Source: CAD feature listing. Evaluate the final solid. Frame: model axes, mm. A direction names the side the tool comes from. Coordinates: 2 decimals unless noted, no trailing zeros. Write each loop counter-clockwise with the first axis right and the second up, starting at its lowest first coordinate (ties: lowest second). Pieces come first, ordered by that corner, then holes. Notation, with made-up numbers: (3.5, 64.5) - (7.5, 64.5) arc R15 cw to (7.5, 78.5) - close; hole circle Ø5 at (-6.75, -15.75). An arc over 180 degrees is marked (long way). One line per question, with ' | ' between items. Start each with the question number.
Q1. Contact query for flat-ended pins moving along their axis: P1, Ø2, axis at x = -22.5, z = 9.5, coming from the -Y side; P2, Ø0.9, axis at x = -8.5, z = -1.5, coming from the +Y side; P3, Ø1.5, axis at x = 22.5, z = -1.5, coming from the -Y side; P4, Ø3.5, axis at x = 4, y = 24, coming from the +Z side. Output: stop coordinate, or through.
Q2. Draft query along X for faces 1 (the face through (-65, 1, -3)), 2 (the face through (-57.09, 12.25, -0.77)). Return one class per face: +X half, -X half, draft (parallel to the pull), parting line (faces both ways), or undercut.
Q3. Cut plane A-A, the plane z = 9. Return loops of the section in (x, y), plus the area to 3 significant figures.
Q4. Cut plane D-D, the plane y = 29. Return loops of the section in (x, z).
Q5. Cut plane B-B, the plane x = 4. Return loops of the section in (y, z).
Q6. Access query for faces 3 (the face through (-5.04, -16.49, -0.77)), 4 (the face through (-168, 0, 2.9)), 5 (the face through (-76.034, 33.187, 16.306)). Directions: +Z, -Z, +X, -X, +Y, -Y. A direction counts if a zero-diameter tool reaches every point of the face in a straight line with its end or side. Return the directions, or none.
Q7. Line query: line 1 (Y direction, x = 4, z = -1.4); line 2 (Y direction, x = 0, z = 24); line 3 (Z direction, x = -48.5, y = -21.5). Output: solid intervals per line, ascending.
Q8. Cut plane C-C, the plane z = 28. Return loops of the section in (x, y), plus the area to 3 significant figures.
```python
from build123d import *

# Parameters (mm, degrees)
ESBO_O1_R                  = 9.95
ESBO_O1_R_2                = 1.9
ESBO_O1_R_3                = 10
ESBO_O1_R_4                = 2.9
RESSALTO_EXTRUS_O1_DEPTH   = 30.8
ESBO_O1_3_R                = 9.95
ESBO_O1_3_R_2              = 1.9
ESBO_O1_3_R_3              = 10
ESBO_O1_3_R_4              = 2.9
RESSALTO_EXTRUS_O2_DEPTH   = 3
RESSALTO_EXTRUS_O4_DEPTH   = 33.8
CORTE_EXTRUS_O1_DEPTH      = 29.4
ESBO_O1_4_R                = 9.95
ESBO_O1_4_R_2              = 1.9
ESBO_O1_4_R_3              = 10
ESBO_O1_4_R_4              = 2.9
CORTE_EXTRUS_O2_DEPTH      = 31.8
CORTE_EXTRUS_O2_DEPTH_BACK = 4
RESSALTO_EXTRUS_O5_DEPTH   = 30.8
FILETE1_R                  = 10
CORTE_EXTRUS_O3_REACH      = 226.029
ESBO_O5_W                  = 22
ESBO_O5_H                  = 6


with BuildPart() as part:
    # Esboço1 → Ressalto-extrusão1 (new body)
    with BuildSketch(Plane.XY):
        with BuildLine():
            Line((-176.929134073, 19.50886441), (-176.929134073, -21.49113559))
            Line((-176.929134073, -21.49113559), (-5.303716409, -42.772427944))
            ThreePointArc((-5.303716409, -42.772427944), (43.09930295, 0.245122927), (-5.789885285, 42.709334207))
            Line((-5.789885285, 42.709334207), (-176.929134073, 19.50886441))
        make_face()
        with Locations((-44.879134073, -0.99113559)):
            Circle(ESBO_O1_R, mode=Mode.SUBTRACT)
        with Locations((-58.844493002, 12.974223338)):
            Circle(ESBO_O1_R_2, mode=Mode.SUBTRACT)
        with Locations((-97.729134073, -0.99113559)):
            Circle(ESBO_O1_R_3, mode=Mode.SUBTRACT)
        with Locations((-58.844493002, -14.956494518)):
            Circle(ESBO_O1_R_2, mode=Mode.SUBTRACT)
        with Locations((4, 24)):
            Circle(ESBO_O1_R_4, mode=Mode.SUBTRACT)
        with BuildLine():
            Line((22.160394843, 16.45886441), (24.010394843, 16.45886441))
            ThreePointArc((24.010394843, 16.45886441), (26.010394843, 14.45886441), (24.010394843, 12.45886441))
            Line((24.010394843, 12.45886441), (22.160394843, 12.45886441))
            ThreePointArc((22.160394843, 12.45886441), (20.160394843, 14.45886441), (22.160394843, 16.45886441))
        make_face(mode=Mode.SUBTRACT)
        with Locations((-30.913775145, -14.956494518)):
            Circle(ESBO_O1_R_2, mode=Mode.SUBTRACT)
        with BuildLine():
            Line((-7.039605157, -18.44113559), (-8.889605157, -18.44113559))
            ThreePointArc((-8.889605157, -18.44113559), (-10.889605157, -16.44113559), (-8.889605157, -14.44113559))
            Line((-8.889605157, -14.44113559), (-7.039605157, -14.44113559))
            ThreePointArc((-7.039605157, -14.44113559), (-5.039605157, -16.44113559), (-7.039605157, -18.44113559))
        make_face(mode=Mode.SUBTRACT)
        with BuildLine():
            Line((24.010394843, -18.44113559), (22.160394843, -18.44113559))
            ThreePointArc((22.160394843, -18.44113559), (20.160394843, -16.44113559), (22.160394843, -14.44113559))
            Line((22.160394843, -14.44113559), (24.010394843, -14.44113559))
            ThreePointArc((24.010394843, -14.44113559), (26.010394843, -16.44113559), (24.010394843, -18.44113559))
        make_face(mode=Mode.SUBTRACT)
        with Locations((-30.913775145, 12.974223338)):
            Circle(ESBO_O1_R_2, mode=Mode.SUBTRACT)
        with BuildLine():
            ThreePointArc((-0.025, -11.375), (-11.4, 0), (-0.025, 11.375))
            Line((-0.025, 11.375), (0.025, 11.375))
            ThreePointArc((0.025, 11.375), (11.4, 0), (0.025, -11.375))
            Line((0.025, -11.375), (-0.025, -11.375))
        make_face(mode=Mode.SUBTRACT)
        with BuildLine():
            ThreePointArc((-8.889605157, 12.45886441), (-10.889605157, 14.45886441), (-8.889605157, 16.45886441))
            Line((-8.889605157, 16.45886441), (-7.039605157, 16.45886441))
            ThreePointArc((-7.039605157, 16.45886441), (-5.039605157, 14.45886441), (-7.039605157, 12.45886441))
            Line((-7.039605157, 12.45886441), (-8.889605157, 12.45886441))
        make_face(mode=Mode.SUBTRACT)
    extrude(amount=RESSALTO_EXTRUS_O1_DEPTH)

    # Esboço1<3> → Ressalto-extrusão2 (add)
    with BuildSketch(Plane.XY):
        with BuildLine():
            Line((-176.929134073, 19.50886441), (-176.929134073, -21.49113559))
            Line((-176.929134073, -21.49113559), (-5.303716409, -42.772427944))
            ThreePointArc((-5.303716409, -42.772427944), (43.09930295, 0.245122927), (-5.789885285, 42.709334207))
            Line((-5.789885285, 42.709334207), (-176.929134073, 19.50886441))
        make_face()
        with Locations((-44.879134073, -0.99113559)):
            Circle(ESBO_O1_3_R, mode=Mode.SUBTRACT)
        with Locations((-58.844493002, 12.974223338)):
            Circle(ESBO_O1_3_R_2, mode=Mode.SUBTRACT)
        with Locations((-97.729134073, -0.99113559)):
            Circle(ESBO_O1_3_R_3, mode=Mode.SUBTRACT)
        with Locations((-58.844493002, -14.956494518)):
            Circle(ESBO_O1_3_R_2, mode=Mode.SUBTRACT)
        with Locations((4, 24)):
            Circle(ESBO_O1_3_R_4, mode=Mode.SUBTRACT)
        with BuildLine():
            Line((22.160394843, 16.45886441), (24.010394843, 16.45886441))
            ThreePointArc((24.010394843, 16.45886441), (26.010394843, 14.45886441), (24.010394843, 12.45886441))
            Line((24.010394843, 12.45886441), (22.160394843, 12.45886441))
            ThreePointArc((22.160394843, 12.45886441), (20.160394843, 14.45886441), (22.160394843, 16.45886441))
        make_face(mode=Mode.SUBTRACT)
        with Locations((-30.913775145, -14.956494518)):
            Circle(ESBO_O1_3_R_2, mode=Mode.SUBTRACT)
        with BuildLine():
            Line((-7.039605157, -18.44113559), (-8.889605157, -18.44113559))
            ThreePointArc((-8.889605157, -18.44113559), (-10.889605157, -16.44113559), (-8.889605157, -14.44113559))
            Line((-8.889605157, -14.44113559), (-7.039605157, -14.44113559))
            ThreePointArc((-7.039605157, -14.44113559), (-5.039605157, -16.44113559), (-7.039605157, -18.44113559))
        make_face(mode=Mode.SUBTRACT)
        with BuildLine():
            Line((24.010394843, -18.44113559), (22.160394843, -18.44113559))
            ThreePointArc((22.160394843, -18.44113559), (20.160394843, -16.44113559), (22.160394843, -14.44113559))
            Line((22.160394843, -14.44113559), (24.010394843, -14.44113559))
            ThreePointArc((24.010394843, -14.44113559), (26.010394843, -16.44113559), (24.010394843, -18.44113559))
        make_face(mode=Mode.SUBTRACT)
        with Locations((-30.913775145, 12.974223338)):
            Circle(ESBO_O1_3_R_2, mode=Mode.SUBTRACT)
        with BuildLine():
            ThreePointArc((-0.025, -11.375), (-11.4, 0), (-0.025, 11.375))
            Line((-0.025, 11.375), (0.025, 11.375))
            ThreePointArc((0.025, 11.375), (11.4, 0), (0.025, -11.375))
            Line((0.025, -11.375), (-0.025, -11.375))
        make_face(mode=Mode.SUBTRACT)
        with BuildLine():
            ThreePointArc((-8.889605157, 12.45886441), (-10.889605157, 14.45886441), (-8.889605157, 16.45886441))
            Line((-8.889605157, 16.45886441), (-7.039605157, 16.45886441))
            ThreePointArc((-7.039605157, 16.45886441), (-5.039605157, 14.45886441), (-7.039605157, 12.45886441))
            Line((-7.039605157, 12.45886441), (-8.889605157, 12.45886441))
        make_face(mode=Mode.SUBTRACT)
    extrude(amount=-RESSALTO_EXTRUS_O2_DEPTH)

    # Esboço4 → Ressalto-extrusão4 (add, through all)
    with BuildSketch(Plane(origin=(0, 0, -3), x_dir=(-1, 0, 0), z_dir=(0, 0, -1))):
        with BuildLine():
            Line((5.549828539, -44.757227385), (178.929134073, -23.258455586))
            Line((178.929134073, -23.258455586), (178.929134073, 21.256028837))
            Line((178.929134073, 21.256028837), (6.058557456, 44.691205864))
            ThreePointArc((6.058557456, 44.691205864), (-45.099270604, 0.25649754), (5.549828539, -44.757227385))
        make_face()
    extrude(amount=-RESSALTO_EXTRUS_O4_DEPTH)

    # Esboço2 → Corte-extrusão1 (cut)
    with BuildSketch(Plane.XY.offset(30.8)):
        with BuildLine():
            Line((-5.789885285, 42.709334207), (-176.929134073, 19.50886441))
            Line((-176.929134073, 19.50886441), (-176.929134073, -21.49113559))
            Line((-176.929134073, -21.49113559), (-5.303716409, -42.772427944))
            ThreePointArc((-5.303716409, -42.772427944), (43.09930295, 0.245122927), (-5.789885285, 42.709334207))
        make_face()
    extrude(amount=-CORTE_EXTRUS_O1_DEPTH, mode=Mode.SUBTRACT)

    # Esboço1<4> → Corte-extrusão2 (cut, two sides)
    with BuildSketch(Plane.XY) as corte_extrus_o2_sk:
        with Locations((-44.879134073, -0.99113559)):
            Circle(ESBO_O1_4_R)
        with Locations((-30.913775145, 12.974223338)):
            Circle(ESBO_O1_4_R_2)
        with Locations((-58.844493002, -14.956494518)):
            Circle(ESBO_O1_4_R_2)
        with Locations((-30.913775145, -14.956494518)):
            Circle(ESBO_O1_4_R_2)
        with Locations((-58.844493002, 12.974223338)):
            Circle(ESBO_O1_4_R_2)
        with Locations((-97.729134073, -0.99113559)):
            Circle(ESBO_O1_4_R_3)
        with Locations((4, 24)):
            Circle(ESBO_O1_4_R_4)
        with BuildLine():
            Line((-0.025, 11.375), (0.025, 11.375))
            ThreePointArc((0.025, 11.375), (11.4, 0), (0.025, -11.375))
            Line((0.025, -11.375), (-0.025, -11.375))
            ThreePointArc((-0.025, -11.375), (-11.4, 0), (-0.025, 11.375))
        make_face()
        with BuildLine():
            Line((22.160394843, 16.45886441), (24.010394843, 16.45886441))
            ThreePointArc((24.010394843, 16.45886441), (26.010394843, 14.45886441), (24.010394843, 12.45886441))
            Line((24.010394843, 12.45886441), (22.160394843, 12.45886441))
            ThreePointArc((22.160394843, 12.45886441), (20.160394843, 14.45886441), (22.160394843, 16.45886441))
        make_face()
        with BuildLine():
            Line((-8.889605157, 16.45886441), (-7.039605157, 16.45886441))
            ThreePointArc((-7.039605157, 16.45886441), (-5.039605157, 14.45886441), (-7.039605157, 12.45886441))
            Line((-7.039605157, 12.45886441), (-8.889605157, 12.45886441))
            ThreePointArc((-8.889605157, 12.45886441), (-10.889605157, 14.45886441), (-8.889605157, 16.45886441))
        make_face()
        with BuildLine():
            Line((22.160394843, -18.44113559), (24.010394843, -18.44113559))
            ThreePointArc((24.010394843, -18.44113559), (26.010394843, -16.44113559), (24.010394843, -14.44113559))
            Line((24.010394843, -14.44113559), (22.160394843, -14.44113559))
            ThreePointArc((22.160394843, -14.44113559), (20.160394843, -16.44113559), (22.160394843, -18.44113559))
        make_face()
        with BuildLine():
            Line((-8.889605157, -18.44113559), (-7.039605157, -18.44113559))
            ThreePointArc((-7.039605157, -18.44113559), (-5.039605157, -16.44113559), (-7.039605157, -14.44113559))
            Line((-7.039605157, -14.44113559), (-8.889605157, -14.44113559))
            ThreePointArc((-8.889605157, -14.44113559), (-10.889605157, -16.44113559), (-8.889605157, -18.44113559))
        make_face()
    extrude(amount=CORTE_EXTRUS_O2_DEPTH, mode=Mode.SUBTRACT)
    extrude(corte_extrus_o2_sk.sketch, amount=-CORTE_EXTRUS_O2_DEPTH_BACK, mode=Mode.SUBTRACT)

    # Esboço1<5> → Ressalto-extrusão5 (add, through all)
    with BuildSketch(Plane.XY):
        Polygon((-156.929134073, 22.220161785), (-176.929134073, 19.50886441), (-176.929134073, -21.49113559), (-156.929134073, -23.971105357), align=None)
    extrude(amount=RESSALTO_EXTRUS_O5_DEPTH)

    # Filete1
    filete1_edges = [part.edges().sort_by_distance(p)[0] for p in [
        (-156.929134073, -23.971105357, 16.1),
        (-156.929134073, 22.220161785, 16.1),
    ]]
    fillet(filete1_edges, radius=FILETE1_R)

    # Esboço5 → Corte-extrusão3 (cut, up to next)
    with BuildSketch(Plane.ZY.offset(178.929134073), mode=Mode.PRIVATE) as corte_extrus_o3_sk1:
        with Locations((13.9, 0)):
            Rectangle(ESBO_O5_W, ESBO_O5_H)
    corte_extrus_o3_tool1 = extrude(corte_extrus_o3_sk1.sketch, amount=-CORTE_EXTRUS_O3_REACH, mode=Mode.PRIVATE) & part.part
    add(corte_extrus_o3_tool1.solids().sort_by_distance((-178.929134, 0, 13.9))[0], mode=Mode.SUBTRACT)


solid = part.part
```
Reply:
1) P1: stops at y = -42.78 | P2: stops at y = 44.42 | P3: stops at y = -39.51 | P4: passes through
2) face 1: draft | face 2: undercut
3) outline: (-178.93, -23.26) - (-5.55, -44.76) arc R45.1 ccw (long way) to (-6.06, 44.69) - (-178.93, 21.26) - (-178.93, 3) - (-156.93, 3) - (-156.93, 13.48) arc R10 cw to (-148.27, 23.39) - (-5.79, 42.71) arc R43.1 cw (long way) to (-5.3, -42.77) - (-148.16, -25.06) arc R10 cw to (-156.93, -15.13) - (-156.93, -3) - (-178.93, -3) - close | area: 1,850 mm^2
4) outline: (-121.81, -3) - (34.54, -3) - (34.54, 30.8) - (31.88, 30.8) - (31.88, 1.4) - (-106.92, 1.4) - (-106.92, 30.8) - (-121.81, 30.8) - close
5) outline: (-44.92, -3) - (-10.66, -3) - (-10.66, 1.4) - (-42.91, 1.4) - (-42.91, 30.8) - (-44.92, 30.8) - close; (10.66, -3) - (21.1, -3) - (21.1, 1.4) - (10.66, 1.4) - close; (26.9, -3) - (44.92, -3) - (44.92, 30.8) - (42.91, 30.8) - (42.91, 1.4) - (26.9, 1.4) - close
6) face 3: +Z, -Z | face 4: -X | face 5: +Z
7) line 1: y = -44.92 to -10.66, 10.66 to 21.1, 26.9 to 44.92 | line 2: y = -45.1 to -43.1, 43.1 to 45.1 | line 3: z = -3 to 1.4
8) outline: (-178.93, -23.26) - (-5.55, -44.76) arc R45.1 ccw (long way) to (-6.06, 44.69) - (-178.93, 21.26) - close; hole (-156.93, -15.13) arc R10 ccw to (-148.16, -25.06) - (-5.3, -42.77) arc R43.1 ccw (long way) to (-5.79, 42.71) - (-148.27, 23.39) arc R10 ccw to (-156.93, 13.48) - close | area: 1,980 mm^2
